from build123d import *

# Parameters (mm, degrees)
F0_R     = 14.25
F0_R_2   = 2.5
F1_DEPTH = 16
F2_DEPTH = 19
F3_R     = 77.5
F4_DEPTH = 6
F5_R     = 4.15
F6_DEPTH = 4


with BuildPart() as f1:
    # F0 (on Top) → F1 (new body)
    with BuildSketch(Plane.XY):
        Circle(F0_R)
        Circle(F0_R_2, mode=Mode.SUBTRACT)
    extrude(amount=F1_DEPTH)

    # F0 (on Top) → F2 (join)
    with BuildSketch(Plane.XY):
        Circle(F0_R_2)
    extrude(amount=F2_DEPTH)

    # F3 (on face) → F4 (join)
    with BuildSketch(Plane.XY.offset(16)):
        Circle(F3_R)
    extrude(amount=F4_DEPTH)

    # F5 (on face) → F6 (join)
    with BuildSketch(Plane(origin=(0, 0, 0), x_dir=(1, 0, 0), z_dir=(0, 0, -1))):
        Circle(F5_R)
    extrude(amount=F6_DEPTH)


solid = f1.part
Source: CAD feature listing. Evaluate the final solid. Frame: model axes, mm. A direction names the side the tool comes from. Round coordinates to 2 decimals unless told otherwise and drop trailing zeros. Order: outer loops, then holes, each group sorted by start corner. A loop starts at its lowest first (then second) coordinate and runs counter-clockwise, first axis right, second up. Notation, with made-up numbers: (61, -21.5) - (76, -21.5) arc R21 ccw to (76, 8.5) - close; hole circle Ø9 at (-15.75, -4). An arc over 180 degrees is marked (long way). Use a Markdown table: item, result. Add a question column.
1. Section query D-D (y = -64.5). Return the cut outline in (x, z).
2. Section query A-A (y = 0). Return the cut outline in (x, z), then the cut area to 3 significant figures.
3. First-contact query: pin 1 (2 mm diameter, centred on x = -41.5, y = -37.5, fed in from -Z); pin 2 (3 mm diameter, centred on y = 1, z = 7.5, fed in from +X); pin 3 (10 mm diameter, centred on y = -54.5, z = 10, fed in from -X); pin 4 (2 mm diameter, centred on x = -9, z = 5, fed in from -Y). Flat tips, straight axial feed; report the tip coordinate or a pass-through.
4. Section query C-C (z = 4.75). Return the cut outline in (x, y), then the cut area to 3 significant figures.
5. Line query: probe 1 along Z at (x, y) = (-38, 35.5); probe 2 along Y at (x, z) = (-10.5, 13.25); probe 3 along Y at (x, z) = (-63, 19.5). Output: solid intervals per line, ascending.
6. Set-up query: faces 1 (the flat face through (-3.4, -3, 0)), 2 (the flat face through (0, 0, -4)). Return all of +Z, -Z, +X, -X, +Y, -Y with unobstructed straight access to the full face (end or side cutting, diameter ignored); none if empty.
Derived:
| question | item | result |
|---|---|---|
| 1 | outline | (-42.97, 16) - (42.97, 16) - (42.97, 22) - (-42.97, 22) - close |
| 2 | outline | (-77.5, 16) - (-14.25, 16) - (-14.25, 0) - (-4.15, 0) - (-4.15, -4) - (4.15, -4) - (4.15, 0) - (14.25, 0) - (14.25, 16) - (77.5, 16) - (77.5, 22) - (-77.5, 22) - close |
| 2 | area | 1,420 mm2 |
| 3 | pin 1 | z = 16 |
| 3 | pin 2 | x = 14.25 |
| 3 | pin 3 | through |
| 3 | pin 4 | y = -11.79 |
| 4 | outline | circle Ø28.5 at (0, 0) |
| 4 | area | 638 mm2 |
| 5 | probe 1 | 16 to 22 |
| 5 | probe 2 | -9.63 to 9.63 |
| 5 | probe 3 | -45.14 to 45.14 |
| 6 | face 1 | -Z |
| 6 | face 2 | -Z, +X, -X, +Y, -Y |
